The model under review builds one solid part; all positions refer to its coordinate system, in mm. Face numbers are marked on the shaded views. Round coordinates to 2 decimals unless told otherwise and drop trailing zeros. Loops run counter-clockwise (first coordinate to the right, second up) from the corner with the lowest first, then second, coordinate; pieces in that order, holes last. Notation, with made-up numbers: (41.25, -24.5) -> (54.25, -24.5) arc R30 ccw to (54.25, 8.5) -> close; hole circle Ø10 at (82, -30). An arc over 180 degrees is marked (long way). Use a Markdown table: item, result. Add a question column.
1) Consider section C-C on z = -4.75. Give the boundary of the cut face in (x, y).
2) Insertion check: pin 1 (7 mm diameter, centred on x = 0, z = 0, fed in from +Y); pin 2 (1 mm diameter, centred on x = 3, y = 11, fed in from +Z); pin 3 (2 mm diameter, centred on x = -4, y = 8, fed in from -Z); pin 4 (4 mm diameter, centred on y = 11.5, z = 3.5, fed in from -X). Each pin has a flat end and moves straight along its axis. Give the tip position at first contact, or say it passes through.
3) Wall thickness on probe 1 along Z at (x, y) = (0, 8.25); probe 2 along Z at (x, y) = (2.25, 10): over which ranges is each line inside the solid? List them lowest first.
4) Consider section A-A on x = 0. Give the boundary of the cut face in (y, z).
5) Consider section B-B on z = 0. Give the boundary of the cut face in (x, y).
6) Mouldability with a two-part tool opening along X and no side actions: class the marked faces 1, 2, 3 and 4 as released by +X, released by -X, zero draft, split by the parting line, or undercut.
Autodesk Inventor part; units mm, degrees
ref_plane "Work Plane7" through (0, 6, 0) normal (0, 1, 0) x (1, 0, 0)
ref_plane "YZ Plane" through (0, 0, 0) normal (1, 0, 0) x (0, 1, 0)
ref_plane "XZ Plane" through (0, 0, 0) normal (0, 1, 0) x (-1, 0, 0)
ref_plane "Work Plane7" through (0, 6, 0) normal (0, 1, 0) x (1, 0, 0)
sketch "Sketch2" plane through (0, 6, 0) normal (0, 1, 0) x (1, 0, 0)
  line L0 (0.7, 6) -> (0.7, 5.9)
  line L1 (-0.7, 6) -> (-0.7, 5.9)
  arc A0 (-0.7, 5.9) -> (0.7, 5.9) centre (0, 5.9) ccw
  line L2 (-1.1884, 5.9227) -> (-1.1575, 5.8275)
  line L3 (-2.5198, 5.49) -> (-2.4889, 5.3949)
  arc A1 (-2.4889, 5.3949) -> (-1.1575, 5.8275) centre (-1.8232, 5.6112) ccw
  line L4 (-2.9604, 5.2656) -> (-2.9016, 5.1846)
  line L5 (-4.093, 4.4427) -> (-4.0342, 4.3618)
  arc A2 (-4.0342, 4.3618) -> (-2.9016, 5.1846) centre (-3.4679, 4.7732) ccw
  line L6 (-4.4427, 4.093) -> (-4.3618, 4.0342)
  line L7 (-5.2656, 2.9604) -> (-5.1846, 2.9016)
  arc A3 (-5.1846, 2.9016) -> (-4.3618, 4.0342) centre (-4.7732, 3.4679) ccw
  line L8 (-5.49, 2.5198) -> (-5.3949, 2.4889)
  line L9 (-5.9227, 1.1884) -> (-5.8275, 1.1575)
  arc A4 (-5.8275, 1.1575) -> (-5.3949, 2.4889) centre (-5.6112, 1.8232) ccw
  line L10 (-6, 0.7) -> (-5.9, 0.7)
  line L11 (-6, -0.7) -> (-5.9, -0.7)
  arc A5 (-5.9, -0.7) -> (-5.9, 0.7) centre (-5.9, 0) ccw
  line L12 (-5.9227, -1.1884) -> (-5.8275, -1.1575)
  line L13 (-5.49, -2.5198) -> (-5.3949, -2.4889)
  arc A6 (-5.3949, -2.4889) -> (-5.8275, -1.1575) centre (-5.6112, -1.8232) ccw
  line L14 (-5.2656, -2.9604) -> (-5.1846, -2.9016)
  line L15 (-4.4427, -4.093) -> (-4.3618, -4.0342)
  arc A7 (-4.3618, -4.0342) -> (-5.1846, -2.9016) centre (-4.7732, -3.4679) ccw
  line L16 (-4.093, -4.4427) -> (-4.0342, -4.3618)
  line L17 (-2.9604, -5.2656) -> (-2.9016, -5.1846)
  arc A8 (-2.9016, -5.1846) -> (-4.0342, -4.3618) centre (-3.4679, -4.7732) ccw
  line L18 (-2.5198, -5.49) -> (-2.4889, -5.3949)
  line L19 (-1.1884, -5.9227) -> (-1.1575, -5.8275)
  arc A9 (-1.1575, -5.8275) -> (-2.4889, -5.3949) centre (-1.8232, -5.6112) ccw
  line L20 (-0.7, -6) -> (-0.7, -5.9)
  line L21 (0.7, -6) -> (0.7, -5.9)
  arc A10 (0.7, -5.9) -> (-0.7, -5.9) centre (0, -5.9) ccw
  line L22 (1.1884, -5.9227) -> (1.1575, -5.8275)
  line L23 (2.5198, -5.49) -> (2.4889, -5.3949)
  arc A11 (2.4889, -5.3949) -> (1.1575, -5.8275) centre (1.8232, -5.6112) ccw
  line L24 (2.9604, -5.2656) -> (2.9016, -5.1846)
  line L25 (4.093, -4.4427) -> (4.0342, -4.3618)
  arc A12 (4.0342, -4.3618) -> (2.9016, -5.1846) centre (3.4679, -4.7732) ccw
  line L26 (4.4427, -4.093) -> (4.3618, -4.0342)
  line L27 (5.2656, -2.9604) -> (5.1846, -2.9016)
  arc A13 (5.1846, -2.9016) -> (4.3618, -4.0342) centre (4.7732, -3.4679) ccw
  line L28 (5.49, -2.5198) -> (5.3949, -2.4889)
  line L29 (5.9227, -1.1884) -> (5.8275, -1.1575)
  arc A14 (5.8275, -1.1575) -> (5.3949, -2.4889) centre (5.6112, -1.8232) ccw
  line L30 (6, -0.7) -> (5.9, -0.7)
  line L31 (6, 0.7) -> (5.9, 0.7)
  arc A15 (5.9, 0.7) -> (5.9, -0.7) centre (5.9, 0) ccw
  line L32 (5.9227, 1.1884) -> (5.8275, 1.1575)
  line L33 (5.49, 2.5198) -> (5.3949, 2.4889)
  arc A16 (5.3949, 2.4889) -> (5.8275, 1.1575) centre (5.6112, 1.8232) ccw
  line L34 (5.2656, 2.9604) -> (5.1846, 2.9016)
  line L35 (4.4427, 4.093) -> (4.3618, 4.0342)
  arc A17 (4.3618, 4.0342) -> (5.1846, 2.9016) centre (4.7732, 3.4679) ccw
  line L36 (4.093, 4.4427) -> (4.0342, 4.3618)
  line L37 (2.9604, 5.2656) -> (2.9016, 5.1846)
  arc A18 (2.9016, 5.1846) -> (4.0342, 4.3618) centre (3.4679, 4.7732) ccw
  line L38 (2.5198, 5.49) -> (2.4889, 5.3949)
  line L39 (1.1884, 5.9227) -> (1.1575, 5.8275)
  arc A19 (1.1575, 5.8275) -> (2.4889, 5.3949) centre (1.8232, 5.6112) ccw
  line L40 (-2.9604, 5.2656) -> (-2.5198, 5.49)
  line L41 (-1.1884, 5.9227) -> (-0.7, 6)
  line L42 (0.7, 6) -> (1.1884, 5.9227)
  line L43 (2.5198, 5.49) -> (2.9604, 5.2656)
  line L44 (4.093, 4.4427) -> (4.4427, 4.093)
  line L45 (5.2656, 2.9604) -> (5.49, 2.5198)
  line L46 (5.9227, 1.1884) -> (6, 0.7)
  line L47 (6, -0.7) -> (5.9227, -1.1884)
  line L48 (5.2656, -2.9604) -> (5.49, -2.5198)
  line L49 (4.4427, -4.093) -> (4.093, -4.4427)
  line L50 (2.9604, -5.2656) -> (2.5198, -5.49)
  line L51 (1.1884, -5.9227) -> (0.7, -6)
  line L52 (-0.7, -6) -> (-1.1884, -5.9227)
  line L53 (-2.5198, -5.49) -> (-2.9604, -5.2656)
  line L54 (-4.093, -4.4427) -> (-4.4427, -4.093)
  line L55 (-5.49, -2.5198) -> (-5.2656, -2.9604)
  line L56 (-5.9227, -1.1884) -> (-6, -0.7)
  line L57 (-6, 0.7) -> (-5.9227, 1.1884)
  line L58 (-5.49, 2.5198) -> (-5.2656, 2.9604)
  line L59 (-4.4427, 4.093) -> (-4.093, 4.4427)
  point P0 (0, 0)
  point P1 (-5.9, 0)
  dimension "d15" = 0.1
  dimension "d16" = 0.7
  dimension "d17" = 0.1
  dimension "d24" = 360
  dimension "d60" = 5.9
  dimension "d61" = 81
extrude "Extrusion9" add sketch "Sketch2" along normal blind 7.5
sketch "Sketch11" plane through (0, 13.5, 0) normal (0, 1, 0) x (1, 0, 0)
  circle A0 centre (0, 0) radius 4
  dimension "d64" = 8
extrude "Extrusion10" cut sketch "Sketch11" against normal up to next
properties part number "PulleyGT2x20Top" material "Aluminum 6061"
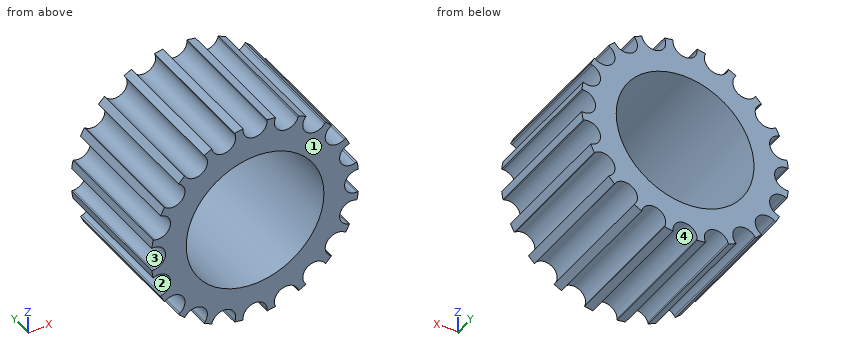
Result set:
| question | item | result |
|---|---|---|
| 1 | outline | (-2.77, 6) -> (2.77, 6) -> (2.77, 13.5) -> (-2.77, 13.5) -> close |
| 2 | pin 1 | through |
| 2 | pin 2 | z = 5.49 |
| 2 | pin 3 | z = -4.44 |
| 2 | pin 4 | x = -5.49 |
| 3 | probe 1 | -5.2 to -4, 4 to 5.2 |
| 3 | probe 2 | -5.06 to -3.31, 3.31 to 5.06 |
| 4 | outline | (6, -5.2) -> (13.5, -5.2) -> (13.5, -4) -> (6, -4) -> close; (6, 4) -> (13.5, 4) -> (13.5, 5.2) -> (6, 5.2) -> close |
| 5 | outline | (-5.2, 6) -> (-4, 6) -> (-4, 13.5) -> (-5.2, 13.5) -> close; (4, 6) -> (5.2, 6) -> (5.2, 13.5) -> (4, 13.5) -> close |
| 6 | face 1 | zero draft |
| 6 | face 2 | undercut |
| 6 | face 3 | released by -X |
| 6 | face 4 | undercut |
